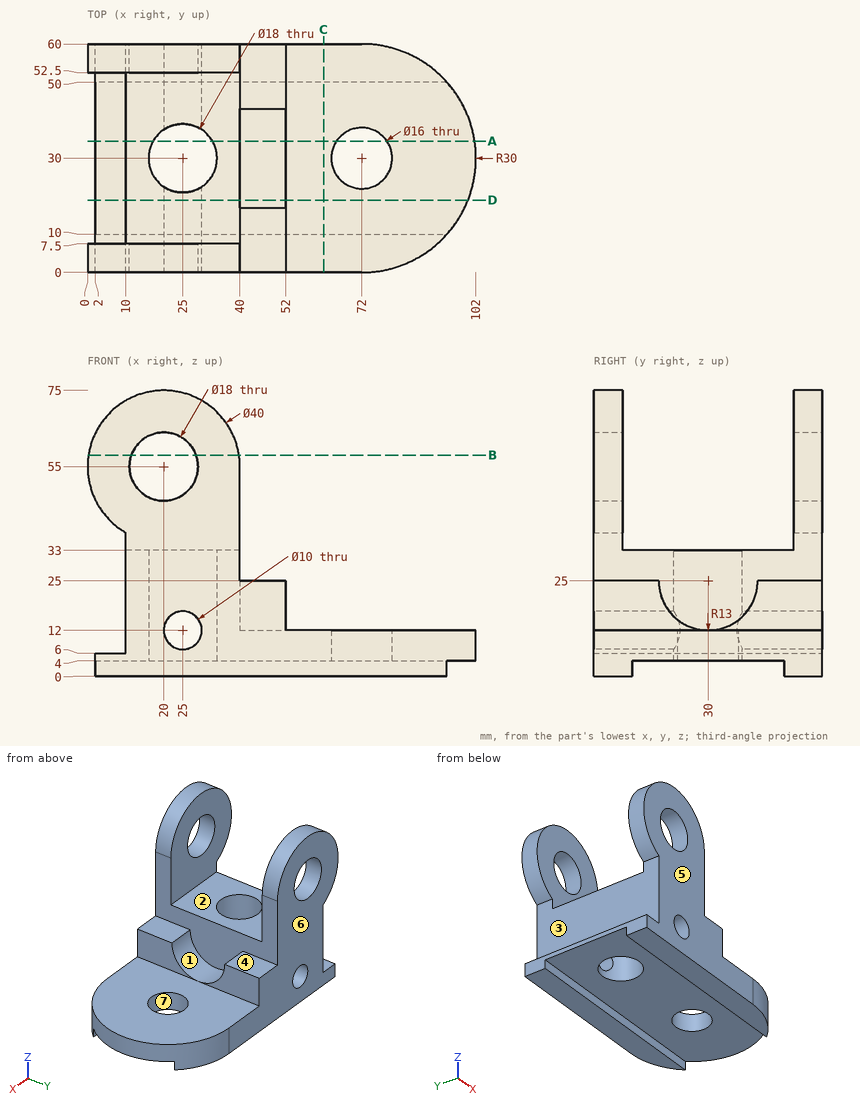
Drawing for the job (mm, zero at the part's lowest x, y, z). A direction names the side the tool comes from. Give positions to 0.01 mm unless a question says otherwise; leave off trailing zeros. Loops run counter-clockwise (first coordinate to the right, second up) from the corner with the lowest first, then second, coordinate; pieces in that order, holes last. Notation, with made-up numbers: (43.5, 77.5) - (49.5, 77.5) arc R22 ccw to (49.5, 88.5) - close; hole circle Ø10 at (-38.75, -17.75). An arc over 180 degrees is marked (long way). Write item = value, one per line. Start each with the question number.
1) Probe probe 1 along Y at (x, z) = (23, 72); probe 2 along Z at (x, y) = (25.5, 5); probe 3 along Z at (x, y) = (25, 54.25). List the from-to ranges inside material, lowest first. Write a range as from..to.
2) Drop flat-ended pins along their axis: pin 1 Ø6 at (x, y) = (66.5, 8.5) entering from +Z; pin 2 Ø3.5 at (x, y) = (46, 54) entering from +Z; pin 3 Ø6 at (x, y) = (83.5, 45) entering from -Z. Give the stop position or say it passes through.
3) Band-saw the part on D-D on y = 19. Give the cut face in (x, z), plus the area to 3 significant figures.
4) Band-saw the part on A-A on y = 34.5. Give the cut face in (x, z), plus the area to 3 significant figures.
5) Pull direction Y, two halves, no side cores. Call the marked faces 4, 5, 6 and 7: +Y half, -Y half, draft (parallel to the pull), parting line (faces both ways), or undercut.
6) Band-saw the part on C-C on x = 62. Give the cut face in (y, z).
7) Band-saw the part on B-B on z = 58. Give the cut face in (x, y).
8) Tool access for the marked faces 1, 2 and 3: list every direction of +Z, -Z, +X, -X, +Y, -Y with a clear straight run to the whole face (end or side of a thin tool).
Final values:
q1.probe_1 = 0..7.5, 52.5..60
q1.probe_2 = 0..7.03, 16.97..47.88, 62.12..74.23
q1.probe_3 = 0..7, 17..47.52, 62.48..74.36
q2.pin_1 = 12
q2.pin_2 = 25
q2.pin_3 = 4
q3.outline = (2, 4) - (99.91, 4) - (99.91, 12) - (52, 12) - (52, 18.07) - (40, 18.07) - (40, 33) - (10, 33) - (10, 6) - (2, 6) - close; hole circle Ø10 at (25, 12)
q3.area = 1,360 mm²
q4.outline = (2, 4) - (17.21, 4) - (17.21, 33) - (10, 33) - (10, 6) - (2, 6) - close; (32.79, 4) - (65.39, 4) - (65.39, 12) - (52, 12) - (52, 12.8) - (40, 12.8) - (40, 33) - (32.79, 33) - close; (78.61, 4) - (101.66, 4) - (101.66, 12) - (78.61, 12) - close
q4.area = 831 mm²
q5.face_4 = draft
q5.face_5 = -Y half
q5.face_6 = +Y half
q5.face_7 = undercut
q6.outline = (0, 0) - (10, 0) - (10, 4) - (50, 4) - (50, 0) - (60, 0) - (60, 12) - (0, 12) - close
q7.outline = (0.23, 0) - (11.51, 0) - (11.51, 7.5) - (0.23, 7.5) - close; (0.23, 52.5) - (11.51, 52.5) - (11.51, 60) - (0.23, 60) - close; (28.49, 0) - (39.77, 0) - (39.77, 7.5) - (28.49, 7.5) - close; (28.49, 52.5) - (39.77, 52.5) - (39.77, 60) - (28.49, 60) - close
q8.face_1 = +Z, +X
q8.face_2 = +Z, +X, -X
q8.face_3 = -X, +Y, -Y
